CAD build for the part. Positions are in the model's coordinates, mm. A direction names the side the tool comes from. Give positions to 0.01 mm unless a question says otherwise; leave off trailing zeros. Loops run counter-clockwise (first coordinate to the right, second up) from the corner with the lowest first, then second, coordinate; pieces in that order, holes last.
Item 1: Probe probe 1 along Z at (x, y) = (23.5, -2); probe 2 along X at (y, z) = (-1.8, 33); probe 3 along X at (y, z) = (-0.55, 43.5). List the from-to ranges inside material, lowest first.
Item 2: Saw through at C-C on y = -0.85. Give the cut face in (x, z), plus the area to 3 significant figures.
Item 3: Drop flat-ended pins along their axis: P1, Ø2, axis at x = 12.5, y = -2, coming from the -Z side; P2, Ø3, axis at x = -22, z = 21, coming from the +Y side; P3, Ø2, axis at y = -2.5, z = 3, coming from the -X side; P4, Ø1.5, axis at x = -25.5, y = -2.5, coming from the +Z side. Give the stop position or say it passes through.
Item 4: Mould opens along Z. For faces 3 (the flat face through (-32, -2, 23.51)), 4 (the cylindrical face through (22.405, -2.129, 66.034)), 5 (the flat face through (-10, -4.318, 18)) say: released by +Z, released by -Z, zero draft, split by the parting line, or undercut.
Item 5: Saw through at D-D on x = -3. Give the cut face in (y, z).
Item 6: Saw through at B-B on z = 2. Give the cut face in (x, y).
Item 7: Which spindle directions (+Z, -Z, +X, -X, +Y, -Y) get a long thin tool onto all of the face, cutting with end or side? Do faces 1 (the flat face through (-10, 0, 18)), 2 (the flat face through (38.658, -2, 36)). Say none if no direction does.
Item 8: Saw through at A-A on x = 19. Give the cut face in (y, z).
from build123d import *

# Parameters (mm, degrees)
F0_R     = 57.924957
F1_DEPTH = 4.318


with BuildPart() as f1:
    # F0 (on Front) → F1 (new body)
    with BuildSketch(Plane.XZ):
        with Locations((-8.735122, 17.191464)):
            Circle(F0_R)
        with BuildLine():
            ThreePointArc((31.223414, 4.553415), (-1.208049, -26.427396), (-33.639513, 4.553415))
            Line((-33.639513, 4.553415), (31.223414, 4.553415))
        make_face(mode=Mode.SUBTRACT)
        Polygon((-45.162439, 23.510488), (-45.162439, 47.299758), (-20.072196, 46.556342), (-20.072196, 23.510488), align=None, mode=Mode.SUBTRACT)
        Polygon((15.054147, 23.510488), (15.054147, 46.556342), (38.657561, 47.299758), (38.657561, 23.510488), align=None, mode=Mode.SUBTRACT)
    extrude(amount=F1_DEPTH)


solid = f1.part
Results below:
1. probe 1: z = -30.94 to -15.02, 4.55 to 23.51, 46.82 to 65.32
1. probe 2: x = -64.46 to -45.16, -20.07 to 15.05, 38.66 to 46.99
1. probe 3: x = -60.34 to -45.16, -20.07 to 15.05, 38.66 to 42.87
2. outline: circle Ø115.85 at (-8.74, 17.19); hole (-45.16, 23.51) - (-20.07, 23.51) - (-20.07, 46.56) - (-45.16, 47.3) - close; hole (-33.64, 4.55) arc R32.47 ccw to (31.22, 4.55) - close; hole (15.05, 23.51) - (38.66, 23.51) - (38.66, 47.3) - (15.05, 46.56) - close
2. area: 7,840 mm2
3. P1: stops at z = -37.08
3. P2: stops at y = 0
3. P3: stops at x = -65.14
3. P4: stops at z = 72.86
4. face 3: undercut
4. face 4: split by the parting line
4. face 5: zero draft
5. outline: (-4.32, -40.45) - (0, -40.45) - (0, -26.38) - (-4.32, -26.38) - close; (-4.32, 4.55) - (0, 4.55) - (0, 74.83) - (-4.32, 74.83) - close
6. outline: (-64.63, -4.32) - (-33.42, -4.32) - (-33.42, 0) - (-64.63, 0) - close; (31.01, -4.32) - (47.16, -4.32) - (47.16, 0) - (31.01, 0) - close
7. face 1: +Z, -Z, +X, -X, +Y
7. face 2: +Y, -Y
8. outline: (-4.32, -33.66) - (0, -33.66) - (0, -19.37) - (-4.32, -19.37) - close; (-4.32, 4.55) - (0, 4.55) - (0, 23.51) - (-4.32, 23.51) - close; (-4.32, 46.68) - (0, 46.68) - (0, 68.04) - (-4.32, 68.04) - close
